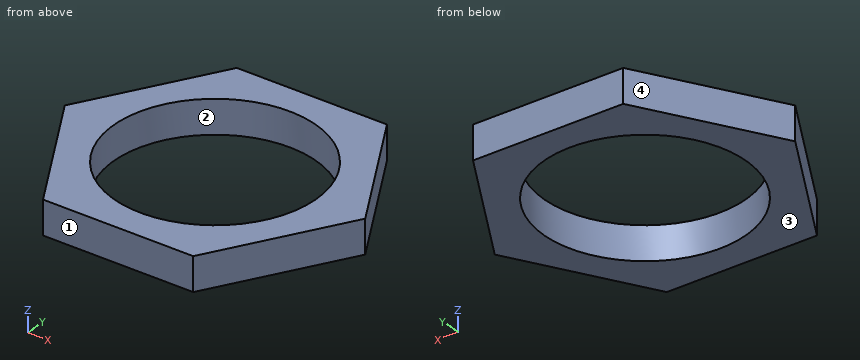
Autodesk Inventor part; units mm, degrees
ref_plane "YZ Plane" through (0, 0, 0) normal (1, 0, 0) x (0, 1, 0)
ref_plane "XZ Plane" through (0, 0, 0) normal (0, 1, 0) x (-1, 0, 0)
ref_plane "XY Plane" through (0, 0, 0) normal (0, 0, 1) x (1, 0, 0)
sketch "Sketch1" plane through (0, 0, 0) normal (0, 0, 1) x (1, 0, 0)
  circle A0 centre (-36.2, 0) radius 6
  circle A1 centre (-36.2, 0) radius 6
  line L0 (-27.2099, 0) -> (-31.705, -7.7856)
  line L1 (-31.705, -7.7856) -> (-40.695, -7.7856)
  line L2 (-40.695, -7.7856) -> (-45.1901, 0)
  line L3 (-45.1901, 0) -> (-40.695, 7.7856)
  line L4 (-40.695, 7.7856) -> (-31.705, 7.7856)
  line L5 (-31.705, 7.7856) -> (-27.2099, 0)
  point P0 (0, 0)
extrude "Extrusion1" add sketch "Sketch1" along normal blind 2
properties part number "NKK_S1AL_mother" material "Stainless Steel"
Design review of the part built by this model. Coordinates are the model's own, in mm. Face numbers are marked on the shaded views. Coordinates: 2 decimals unless noted, no trailing zeros. Order: outer loops, then holes, each group sorted by start corner. A loop starts at its lowest first (then second) coordinate and runs counter-clockwise, first axis right, second up. Notation, with made-up numbers: (18, 12.5) - (70, 12.5) arc R17 ccw to (70, 38.5) - close; hole circle Ø9 at (82.25, 15). An arc over 180 degrees is marked (long way). Answer in a Markdown table with one row per item.
(1) Consider section A-A on x = -36.2. State the section outline as (y, z) points, plus the area to 3 significant figures.
Checked values:
| item | result |
|---|---|
| outline | (-7.79, 0) - (-6, 0) - (-6, 2) - (-7.79, 2) - close; (6, 0) - (7.79, 0) - (7.79, 2) - (6, 2) - close |
| area | 7.14 mm^2 |
(2) Consider section B-B on y = -1.25. State the section outline as (x, z) points, plus the area to 3 significant figures.
Checked values:
| item | result |
|---|---|
| outline | (-44.47, 0) - (-42.07, 0) - (-42.07, 2) - (-44.47, 2) - close; (-30.33, 0) - (-27.93, 0) - (-27.93, 2) - (-30.33, 2) - close |
| area | 9.60 mm^2 |
(3) Consider section C-C on z = 0.7. State the section outline as (x, y) points (3 decimals), plus the area to 3 significant figures.
Checked values:
| item | result |
|---|---|
| outline | (-45.19, 0) - (-40.695, -7.786) - (-31.705, -7.786) - (-27.21, 0) - (-31.705, 7.786) - (-40.695, 7.786) - close; hole circle Ø12 at (-36.2, 0) |
| area | 96.9 mm^2 |
(4) Consider section D-D on x = -30. State the section outline as (y, z) points.
Checked values:
| item | result |
|---|---|
| outline | (-4.83, 0) - (4.83, 0) - (4.83, 2) - (-4.83, 2) - close |
(5) Wall thickness on line 1 along Y through (x, z) = (-36.2, 0.8); line 2 along Y through (x, z) = (-37.75, 0.25); line 3 along X through (y, z) = (-2.5, 1.4): over which ranges is each line inside the solid? List them lowest first. Write a range as from..to.
Checked values:
| item | result |
|---|---|
| line 1 | -7.79..-6, 6..7.79 |
| line 2 | -7.79..-5.8, 5.8..7.79 |
| line 3 | -43.75..-41.65, -30.75..-28.65 |
(6) The part is to be moulded in two halves that separate along Y. For the marked faces 1, 2, 3 and 4, say which applies: released by +Y, released by -Y, zero draft, split by the parting line, or undercut.
Checked values:
| item | result |
|---|---|
| face 1 | released by -Y |
| face 2 | undercut |
| face 3 | zero draft |
| face 4 | released by +Y |
